Geometry: final body of the model. Coordinates: model frame, mm. A direction names the side the tool comes from. Give positions to 0.01 mm unless a question says otherwise; leave off trailing zeros. Order: outer loops, then holes, each group sorted by start corner. A loop starts at its lowest first (then second) coordinate and runs counter-clockwise, first axis right, second up. Notation, with made-up numbers: (-18.75, 51.5) - (0.25, 51.5) arc R10 cw to (0.25, 67.5) - close; hole circle Ø1 at (86.5, 19.25). An arc over 180 degrees is marked (long way). One line per question, with ' | ' between items. Start each with the question number.
Autodesk Inventor part; units mm, degrees
ref_plane "YZ Plane" through (0, 0, 0) normal (1, 0, 0) x (0, 1, 0)
ref_plane "XZ Plane" through (0, 0, 0) normal (0, 1, 0) x (-1, 0, 0)
ref_plane "XY Plane" through (0, 0, 0) normal (0, 0, 1) x (1, 0, 0)
sketch "Sketch1" plane through (0, 0, 0) normal (0, 0, 1) x (1, 0, 0)
  line L0 (0, 0) -> (-5, 0)
  line L1 (-5, 0) -> (-5, -68.15)
  line L2 (-5, -68.15) -> (0, -68.15)
  line L3 (0, -68.15) -> (0, 0)
  line L4 (0, 13.63) -> (0, -81.78)
  line L5 (-6, 0) -> (1, 0)
  dimension "d1" = 68.15
  dimension "d2" = 5
revolve "Shoulder" add sketch "Sketch1" angle 360 about axis through (0, -68.15, 0) along (0, 1, 0)
sketch "Sketch2" plane through (0, 0, 0) normal (0, 1, 0) x (1, 0, 0)
  circle A0 centre (0, 0) radius 5
  circle A1 centre (0, 0) radius 4.76
  dimension "d3" = 9.52
extrude "Shoulder_neck" add sketch "Sketch2" along normal blind 1.85 contours A1
sketch "Sketch3" plane through (0, 1.85, 0) normal (0, 1, 0) x (1, 0, 0)
  circle A0 centre (0, 0) radius 4.76
  circle A1 centre (0, 0) radius 8.1
  dimension "d6" = 16.2
extrude "Head" add sketch "Sketch3" along normal blind 7 contours A0 | A1
sketch "Sketch4" plane through (0, -68.15, 0) normal (0, -1, 0) x (1, 0, 0)
  circle A0 centre (0, 0) radius 5
  circle A1 centre (0, 0) radius 3.09
  dimension "d9" = 6.18
extrude "Thread_neck" add sketch "Sketch4" along normal blind 2.6 contours A1
sketch "Sketch5" plane through (0, -70.75, 0) normal (0, -1, 0) x (1, 0, 0)
  circle A0 centre (0, 0) radius 3.09
  circle A1 centre (0, 0) radius 4
  dimension "d12" = 8
extrude "Thread_shoulder" add sketch "Sketch5" along normal blind 10.4 contours A0 | A1
sketch "Sketch6" plane through (0, 8.85, 0) normal (0, 1, 0) x (1, 0, 0)
  circle A0 centre (0, 0) radius 8.1
  circle A1 centre (0, 0) radius 2.5 construction
  line L0 (-2.5, 1.4434) -> (-2.5, -1.4434)
  line L1 (-2.5, -1.4434) -> (0, -2.8868)
  line L2 (0, -2.8868) -> (2.5, -1.4434)
  line L3 (2.5, -1.4434) -> (2.5, 1.4434)
  line L4 (2.5, 1.4434) -> (0, 2.8868)
  line L5 (0, 2.8868) -> (-2.5, 1.4434)
  dimension "d15" = 5
extrude "Hex" cut sketch "Sketch6" against normal blind 4.2 contours L5 L4 L3 L2 L1 L0
chamfer "Chamfer1" distance 0.24 angle 30 1 edges at (5, 0, 0) measured on face at (-4.8255, 0, -0.7786)
fillet "Fillet1" radius 0.4 1 edges at (-4.76, 1.85, 0)
chamfer "Chamfer2" distance 0.5 angle 30 1 edges at (-8.1, 8.85, 0) measured on face at (7.9951, 6.5167, 1.2993)
chamfer "Chamfer3" distance 0.625 angle 30 1 edges at (-4, -81.15, 0) measured on face at (0.7574, -81.15, 1.0973)
fillet "Fillet2" radius 0.7 1 edges at (-3.09, -68.15, 0)
chamfer "Chamfer7" distance 0.91 angle 30 1 edges at (-4, -70.75, 0) measured on face at (3.6579, -70.75, -0.3191)
thread "Thread"
equation "\"d3\" = Shoulder_neck_dia"
equation "\"d4\" = Shoulder_neck_length"
equation "\"d6\" = Head_diameter"
equation "\"d7\" = Head_height"
equation "\"d9\" = Thread_neck_dia"
equation "\"d10\" = Thread_neck_length"
equation "\"d12\" = Thread_diameter"
equation "\"d13\" = Thread_length - Thread_neck_length"
equation "\"d15\" = Hex_size"
equation "\"d16\" = Hex_length"
equation "\"d18\" = -0.5 * Shoulder_neck_dia + 0.5 * Shoulder_diameter"
equation "\"d64\" = -0.5 * Shoulder_neck_dia + 0.5 * Shoulder_diameter"
equation "\"d21\" = 0.1 * Hex_size"
equation "\"d65\" = 0.1 * Hex_size"
equation "\"d23\" = 0.5 * Thread_pitch"
equation "\"d66\" = 0.5 * Thread_pitch"
equation "\"d25\" = Thread_neck_radius"
equation "\"d60\" = -0.5 * Thread_neck_dia + 0.5 * Thread_diameter"
equation "\"d67\" = -0.5 * Thread_neck_dia + 0.5 * Thread_diameter"
equation "\"Shoulder_neck_dia\" = 9.52"
equation "\"Thread_diameter\" = 8"
equation "\"Thread_length\" = 13"
equation "\"Head_diameter\" = 16.2"
equation "\"Head_height\" = 7"
equation "\"Thread_neck_dia\" = 6.18"
equation "\"Hex_size\" = 5"
equation "\"Hex_length\" = 4.2"
equation "\"Thread_pitch\" = 1.25"
equation "\"Shoulder_neck_length\" = 1.85"
equation "\"Thread_neck_length\" = 2.6"
equation "\"Thread_neck_radius\" = 0.7"
properties part number "SCREW, SHOULDER, P, 12.9, 10MMX70MM" material "Steel, High Strength Low Alloy"
(1) Cut plane A-A, the plane y = -61. Return the cut outline in (x, z).
(2) Pull-direction query (Y, two-part tool) for faces 4 (the flat face through (5, 1.85, 2)), 5 (the cylindrical face through (1.08, -34.62, 4.88)), 6 (the cylindrical face through (1.661, -69.787, -2.605)), 7 (the flat face through (-2, 8.85, -2)); classes: +Y half, -Y half, draft (parallel to the pull), parting line (faces both ways), or undercut.
(3) Material intervals for line 1 along Y through (x, z) = (5.5, 2); line 2 along Y through (x, z) = (3.75, -2.25); line 3 along X through (y, z) = (-63.5, -0.25), sorted ascending. Write a range as from..to.
(4) Access query for faces 1 (the flat face through (1, -68.15, 4)), 2 (the flat face through (0, -81.15, 0)), 3 (the flat face through (-1.267, 6.779, 2.155)). Directions: +Z, -Z, +X, -X, +Y, -Y. A direction counts if a zero-diameter tool reaches every point of the face in a straight line with its end or side. Return the directions, or none.
(5) Contact query for flat-ended pins moving along their axis: P1, Ø5, axis at x = -2.5, y = -46.5, coming from the -Z side; P2, Ø4, axis at y = -42, z = -3.5, coming from the +X side; P3, Ø1.9, axis at x = 0, z = -0.5, coming from the +Y side. Output: stop coordinate, or through.
Results are:
1) outline: circle Ø10 at (0, 0)
2) face 4: -Y half | face 5: draft | face 6: undercut | face 7: +Y half
3) line 1: 1.85..8.85 | line 2: -68.15..8.85 | line 3: -4.99..4.99
4) face 1: none | face 2: +Z, -Z, +X, -X, -Y | face 3: +Y
5) P1: z = -5 | P2: x = 4.77 | P3: y = 4.65
